Autodesk Inventor part; units mm, degrees
ref_plane "YZ Plane" through (0, 0, 0) normal (1, 0, 0) x (0, 1, 0)
ref_plane "XZ Plane" through (0, 0, 0) normal (0, 1, 0) x (-1, 0, 0)
ref_plane "XY Plane" through (0, 0, 0) normal (0, 0, 1) x (1, 0, 0)
sketch "Szkic1" plane through (0, 0, 0) normal (0, 1, 0) x (-1, 0, 0)
  line L0 (16.25, 26.75) -> (-16.25, 26.75)
  line L1 (-16.25, 26.75) -> (-16.25, -26.75)
  line L2 (-16.25, -26.75) -> (16.25, -26.75)
  line L3 (16.25, -26.75) -> (16.25, 26.75)
  point P0 (0, 0)
  point P1 (0, 0)
  point P2 (0, 26.75)
  dimension "d0" = 32.5
  dimension "d1" = 53.5
  dimension "d2" = 26.75
  dimension "d3" = 16.25
extrude "Wyciągnięcie proste1" add sketch "Szkic1" along normal blind 8
sketch "Szkic2" plane through (0, 8, 0) normal (0, 1, 0) x (1, 0, 0)
  line L0 (-16.25, -26.75) -> (16.25, -26.75)
  line L1 (-16.25, 26.75) -> (-16.25, -26.75)
  line L2 (16.25, -26.75) -> (16.25, 26.75)
  line L3 (-16.25, -13.75) -> (-11.45, -13.75)
  line L4 (-11.45, -13.75) -> (-11.45, -10.75)
  line L5 (-11.45, -10.75) -> (-16.25, -10.75)
  line L6 (-16.25, -10.75) -> (-16.25, -13.75)
  line L7 (16.25, -13.75) -> (11.45, -13.75)
  line L8 (11.45, -13.75) -> (11.45, -10.75)
  line L9 (11.45, -10.75) -> (16.25, -10.75)
  line L10 (16.25, -10.75) -> (16.25, -13.75)
  line L11 (-16.25, 23.75) -> (-11.45, 23.75)
  line L12 (-11.45, 23.75) -> (-11.45, 20.75)
  line L13 (-11.45, 20.75) -> (-16.25, 20.75)
  line L14 (-16.25, 20.75) -> (-16.25, 23.75)
  line L15 (16.25, 20.75) -> (11.45, 20.75)
  line L16 (11.45, 20.75) -> (11.45, 23.75)
  line L17 (11.45, 23.75) -> (16.25, 23.75)
  line L18 (16.25, 23.75) -> (16.25, 20.75)
  point P0 (0, 0)
  dimension "d7" = 4.8
  dimension "d8" = 3
  dimension "d9" = 4.8
  dimension "d10" = 3
  dimension "d11" = 4.8
  dimension "d12" = 3
  dimension "d13" = 4.8
  dimension "d14" = 3
  dimension "d15" = 13
  dimension "d16" = 13
  dimension "d17" = 3
  dimension "d18" = 3
extrude "Wyciągnięcie proste2" add sketch "Szkic2" along normal blind 12.7
sketch "Szkic3" plane through (-16.25, 8, 13.75) normal (0, 0, 1) x (1, 0, 0)
  circle A0 centre (2.4, 6.3) radius 1.525
  circle A1 centre (30.1, 6.3) radius 1.525
  line L0 (0, 0) -> (32.5, 0)
  line L1 (4.8, 0) -> (4.8, 12.7)
  line L2 (32.5, 0) -> (32.5, 12.7)
  point P0 (16.25, -8)
  dimension "d21" = 3.05
  dimension "d22" = 3.05
  dimension "d23" = 6.3
  dimension "d24" = 6.3
  dimension "d25" = 2.4
  dimension "d26" = 2.4
sketch "Szkic4" plane through (-16.25, 8, -20.75) normal (0, 0, 1) x (1, 0, 0)
  point P0 (16.25, -8)
sketch "Szkic5" plane through (-11.45, 8, -23.75) normal (0, 0, -1) x (-1, 0, 0)
  circle A0 centre (-25.3, 6.3) radius 1.525
  circle A1 centre (2.4, 6.3) radius 1.525
  line L0 (-27.7, 0) -> (4.8, 0)
  line L1 (-22.9, 0) -> (-22.9, 12.7)
  line L2 (4.8, 0) -> (4.8, 12.7)
  point P0 (-11.45, -8)
  dimension "d27" = 3.05
  dimension "d28" = 3.05
  dimension "d29" = 6.3
  dimension "d30" = 2.4
  dimension "d31" = 2.4
  dimension "d32" = 6.3
extrude "Wyciągnięcie proste3" cut sketch "Szkic3" against normal blind 3
extrude "Wyciągnięcie proste4" cut sketch "Szkic5" against normal blind 3
sketch "Szkic6" plane through (0, 8, 0) normal (0, 1, 0) x (1, 0, 0)
  circle A0 centre (-9.75, 14.75) radius 1.5
  line L0 (16.25, 26.75) -> (-16.25, 26.75)
  line L1 (-16.25, 20.75) -> (-16.25, -10.75)
  circle A1 centre (-9.75, -20.25) radius 1.5
  line L2 (0, 26.75) -> (0, -26.75)
  line L3 (-16.25, -26.75) -> (16.25, -26.75)
  circle A2 centre (9.75, 14.75) radius 1.5
  circle A3 centre (9.75, -20.25) radius 1.5
  point P0 (0, 0)
  dimension "d37" = 3
  dimension "d38" = 12
  dimension "d39" = 6.5
  dimension "d42" = 35
  dimension "d49" = 9.75
extrude "Wyciągnięcie proste5" cut sketch "Szkic6" against normal blind 10
properties part number "Base_to_servo_mount"
Build history of the part. All positions in model axes, mm. A direction names the side the tool comes from. Round coordinates to 2 decimals unless told otherwise and drop trailing zeros. Write each loop counter-clockwise with the first axis right and the second up, starting at its lowest first coordinate (ties: lowest second). Pieces come first, ordered by that corner, then holes. Notation, with made-up numbers: M 3,-21 L 46,-21 A26 ccw 46,2 Z; hole C 28.25,26.25 d2. An arc over 180 degrees is marked long. Answer as a JSON object with one key per item and string values. Group by question number.
(1) Cut at C-C (y = 4). Give the cut face in (x, z), and give its area (3 significant figures).
(2) Which spindle directions (+Z, -Z, +X, -X, +Y, -Y) get a long thin tool onto all of the face, cutting with end or side? Do faces 1 (the flat face through (12, 14, -23.75)), 2 (the flat face through (0, 4, -26.75)), 3 (the flat face through (12, 14, 13.75)), 4 (the flat face through (-12, 14, 10.75)), 5 (the flat face through (11.45, 14, 12)). Say none if no direction does.
(3) Cut at D-D (z = 12). Give the cut face in (x, y) (3 decimals).
(4) Cut at B-B (z = -14.75). Give the cut face in (x, y).
(5) Cut at A-A (x = 9.75). Give the cut face in (y, z), and give its area (3 significant figures).
(6) Mould opens along Y. For faces 6 (the flat face through (-11.45, 14, -22)), 7 (the cylindrical face through (-15, 15.3, 12.3)), 8 (the flat face through (-14, 20.7, 12)) say: pulls with the +Y half, pulls with the -Y half, needs draft (parallel to the pull), parting line crosses it, or undercut.
(7) Flat gauge pins, fed straight in: pin 1 (5.5 mm diameter, centred on x = 14.5, y = 14, fed in from +Z); pin 2 (5 mm diameter, centred on x = 9.75, z = 20.25, fed in from +Y); pin 3 (5 mm diameter, centred on x = 9.75, z = -14.75, fed in from -Y); pin 4 (4 mm diameter, centred on x = -15, y = 15, fed in from -Z). Where does each tip first touch, or does it go through?
(8) Drill centre lines: L1, parallel to Z at x = -9.75, y = 2.25; L2, parallel to X at y = 5.75, z = 20.25; L3, parallel to Y at x = -13.85, z = -22.5 (3 decimals). Where is each one in solid material? Low to high.
Responses:
{
 "1": {"outline": "M -16.25,-26.75 L 16.25,-26.75 L 16.25,26.75 L -16.25,26.75 Z; hole C -9.75,-14.75 d3; hole C -9.75,20.25 d3; hole C 9.75,-14.75 d3; hole C 9.75,20.25 d3", "area": "1,710 mm2"},
 "2": {"face 1": "-Z, +X, -X, +Y", "face 2": "-Z, +X, -X, +Y, -Y", "face 3": "+Z, +X, -X, +Y", "face 4": "+X, -X, +Y", "face 5": "+Z, -Z, +Y"},
 "3": {"outline": "M -16.25,0 L 16.25,0 L 16.25,20.7 L 11.45,20.7 L 11.45,8 L -11.45,8 L -11.45,20.7 L -16.25,20.7 Z; hole C -13.85,14.3 d3.05; hole C 13.85,14.3 d3.05"},
 "4": {"outline": "M -16.25,0 L -11.25,0 L -11.25,8 L -16.25,8 Z; M -8.25,0 L 8.25,0 L 8.25,8 L -8.25,8 Z; M 11.25,0 L 16.25,0 L 16.25,8 L 11.25,8 Z"},
 "5": {"outline": "M 0,-26.75 L 8,-26.75 L 8,-16.25 L 0,-16.25 Z; M 0,-13.25 L 8,-13.25 L 8,18.75 L 0,18.75 Z; M 0,21.75 L 8,21.75 L 8,26.75 L 0,26.75 Z", "area": "380 mm2"},
 "6": {"face 6": "needs draft", "face 7": "undercut", "face 8": "pulls with the +Y half"},
 "7": {"pin 1": "stops at z = 13.75", "pin 2": "stops at y = 8", "pin 3": "stops at y = 0", "pin 4": "stops at z = -23.75"},
 "8": {"L1": "z = -26.75 to -16.25, -13.25 to 18.75, 21.75 to 26.75", "L2": "x = -16.25 to -11.25, -8.25 to 8.25, 11.25 to 16.25", "L3": "y = 0 to 12.775, 15.825 to 20.7"}
}
